The figure shows three views and two pictorial views of one solid part (mm, origin at its lowest corner). Answer the questions. Coordinates: 2 decimals unless noted, no trailing zeros. Write each loop counter-clockwise with the first axis right and the second up, starting at its lowest first coordinate (ties: lowest second). Pieces come first, ordered by that corner, then holes.
Item 1: Each of these flat-tipped pins is pushed along its axis until it touches: P1, Ø8, axis at x = 375, z = 22.5, coming from the -Y side; P2, Ø5, axis at x = 333.5, y = 28, coming from the +Z side; P3, Ø1.5, axis at x = 396.5, z = 21, coming from the -Y side; P4, Ø1.5, axis at y = 26, z = 26.5, coming from the +X side. Where does it stop, or does it pass through?
Item 2: Section A-A (z = 15) is taken. Give the vertices of the cut face in (x, y), then the cut area to 3 significant figures.
Item 3: Section C-C (y = 21) is taken. Give the vertices of the cut face in (x, z).
Item 4: Straight lines are drawn through the part: probe 1 along Y at (x, z) = (543.5, 13.5) (1 decimal); probe 2 along X at (y, z) = (30, 17.5); probe 3 along Z at (x, y) = (183.5, 15.5). For each, find the intervals that lie inside material, in ascending order.
Item 5: Section B-B (x = 182) is taken. Give the vertices of the cut face in (y, z).
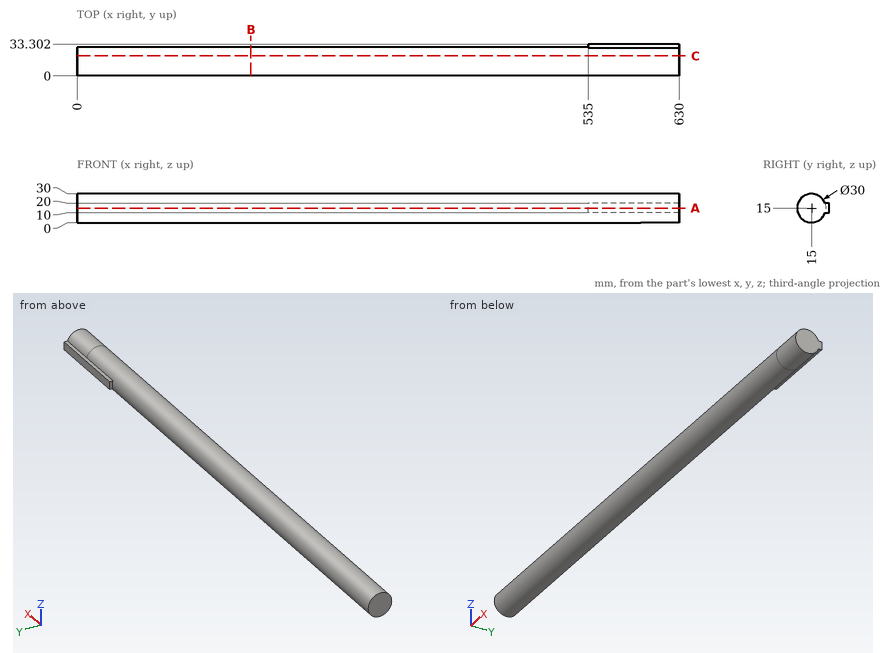
Established:
1. P1: stops at y = 0.41
1. P2: stops at z = 25.71
1. P3: stops at y = 0.95
1. P4: passes through
2. outline: (0, 0) - (630, 0) - (630, 33.3) - (535, 33.3) - (535, 30) - (0, 30) - close
2. area: 19,200 mm2
3. outline: (0, 1.25) - (630, 1.25) - (630, 28.75) - (0, 28.75) - close
4. probe 1: y = 0.1 to 33.3
4. probe 2: x = 535 to 630
4. probe 3: z = 0.01 to 29.99
5. outline: circle Ø30 at (15, 15)
